from build123d import *

# Parameters (mm, degrees)
SKETCH_R             = 1.5
PAD_DEPTH            = 35
PAD001_DEPTH         = 0.5
SKETCH002_R          = 1.5
PAD002_DEPTH         = 19
PAD003_DEPTH         = 0.5
POLARPATTERN_COUNT   = 2
POLARPATTERN_ANGLE   = 90
SKETCH004_R          = 10
PAD004_DEPTH         = 10
SKETCH006_W          = 5.388718
SKETCH006_H          = 19
SKETCH006_W_2        = 5.907516
POCKET_DEPTH         = 5
SKETCH005_W          = 53.248554
SKETCH005_H          = 72.779518
SKETCH005_W_2        = 13.520593
SKETCH005_H_2        = 41.716759
POCKET001_DEPTH      = 10.001
POCKET001_DEPTH_BACK = -10.001


with BuildPart() as part:
    # Sketch → Pad (new body)
    with BuildSketch(Plane.XY):
        Circle(SKETCH_R)
    extrude(amount=PAD_DEPTH)

    # Sketch001 → Pad001 (join, symmetric)
    with BuildSketch(Plane.XZ):
        Polygon((-3.25, 0), (3.25, 0), (3.25, 1.5), (1.083333, 4.5), (3.25, 7.5), (3.25, 9), (-3.25, 9), (-3.25, 7.5), (-1.083333, 4.5), (-3.25, 1.5), align=None)
    extrude(amount=PAD001_DEPTH, both=True)

    # Sketch002 → Pad002 (join)
    with BuildSketch(Plane.XY):
        Circle(SKETCH002_R)
    extrude(amount=-PAD002_DEPTH)

    # Sketch003 → Pad003 (join, symmetric)
    with BuildSketch(Plane.XZ):
        Polygon((-3.4, -19), (3.4, -19), (3.4, -9), (0, 2), (-3.4, -9), align=None)
    pad003 = extrude(amount=PAD003_DEPTH, both=True)

    # PolarPattern: Pad003 ×2 about axis
    polarpattern_axis = Axis((0, 0, 0), (0, 0, 1))
    for i in range(1, POLARPATTERN_COUNT):
        add(pad003.rotate(polarpattern_axis, i * POLARPATTERN_ANGLE / (POLARPATTERN_COUNT - 1)))

    # Sketch004 → Pad004 (join)
    with BuildSketch(Plane.XY.offset(-19)):
        Circle(SKETCH004_R)
    extrude(amount=-PAD004_DEPTH)

    # Sketch006 → Pocket (cut, symmetric)
    with BuildSketch(Plane.YZ):
        with Locations((5.194359, -9.5)):
            Rectangle(SKETCH006_W, SKETCH006_H)
        with Locations((-5.453758, -9.5)):
            Rectangle(SKETCH006_W_2, SKETCH006_H)
    extrude(amount=POCKET_DEPTH, both=True, mode=Mode.SUBTRACT)

    # Sketch005 → Pocket001 (cut, two sides)
    with BuildSketch(Plane.XZ) as pocket001_sk:
        with Locations((-0.717024, -0.672455)):
            Rectangle(SKETCH005_W, SKETCH005_H)
        with Locations((0.133193, -10.244297)):
            Rectangle(SKETCH005_W_2, SKETCH005_H_2, mode=Mode.SUBTRACT)
    extrude(amount=-POCKET001_DEPTH, mode=Mode.SUBTRACT)
    extrude(pocket001_sk.sketch, amount=-POCKET001_DEPTH_BACK, mode=Mode.SUBTRACT)


solid = part.part
Design review of the part built by this model. Coordinates are the model's own, in mm. A direction names the side the tool comes from. Round coordinates to 2 decimals unless told otherwise and drop trailing zeros. Write each loop counter-clockwise with the first axis right and the second up, starting at its lowest first coordinate (ties: lowest second). Pieces come first, ordered by that corner, then holes. Notation, with made-up numbers: (8, -37.5) - (51, -37.5) arc R24 cw to (51, -20.5) - close; hole circle Ø5 at (8, 84). An arc over 180 degrees is marked (long way). Return JSON: item names as keys, results as strings. Group by question number.
Item 1: We need section B-B on x = 0. Write out the cut boundary in (y, z).
Item 2: Machinability: for faces 4 (the face through (2, -0.5, -12)), 5 (the face through (-3.4, 0, -14)), 6 (the face through (0, -2.5, -13)), 7 (the face through (-2, 0.5, 7)), 8 (the face through (0, 2.5, -13)), which of the approach directions +Z, -Z, +X, -X, +Y, -Y give a long, thin tool a straight path to every point of the face, cutting with its end or side? Answer none if there is none.
Item 3: For probe 1 along Z at (x, y) = (0.75, -1.5); probe 2 along Y at (x, z) = (3.25, -12); probe 3 along X at (y, z) = (-9, -20), list the stretches that pass through material, from the lowest coordinate up. Write a range as [from, to].
Item 4: We need section C-C on y = 3.75. Write out the cut boundary in (x, z), and give its area (3 significant figures).
Item 5: We need section A-A on z = -13.5. Write out the cut boundary in (x, y).
Item 6: We need section D-D on z = 1. Write out the cut boundary in (x, y), and give its area (3 significant figures).
Item 7: Insertion check: P1, Ø0.5, axis at x = 0, z = -12, coming from the +Y side; P2, Ø0.6, axis at x = 2.5, z = 7, coming from the +Y side; P3, Ø2, axis at x = 2, z = 6, coming from the -Y side. Each pin has a flat end and moves straight along its axis. Give the tip position at first contact, or say it passes through.
Item 8: The part is to be moulded in two halves that separate along Z. For faces 1 (the face through (2, 0.5, 2)), 2 (the face through (-2, 0, 9)), 3 (the face through (-2.32, -0.01, 2.79)), say which applies: pulls with the +Z half, pulls with the -Z half, needs draft (parallel to the pull), parting line crosses it, or undercut.
Model answer:
{
 "1": {"outline": "(-10, -29) - (10, -29) - (10, -19) - (2.5, -19) - (2.5, -6.09) - (1.5, -2.85) - (1.5, 10.61) - (-1.5, 10.61) - (-1.5, -2.85) - (-2.5, -6.09) - (-2.5, -19) - (-10, -19) - close"},
 "2": {"face 4": "+Z, +X, -Y", "face 5": "+Z, -X, +Y, -Y", "face 6": "+Z, +X, -X, -Y", "face 7": "+Z, -X, +Y", "face 8": "+Z, +X, -X, +Y"},
 "3": {"probe 1": "z = [-29, -19]", "probe 2": "y = [-0.5, 0.5]", "probe 3": "x = [-4.36, 4.36]"},
 "4": {"outline": "(-6.63, -29) - (6.89, -29) - (6.89, -19) - (-6.63, -19) - close", "area": "135 mm²"},
 "5": {"outline": "(-3.4, -0.5) - (-1.41, -0.5) arc R1.5 ccw to (-0.5, -1.41) - (-0.5, -2.5) - (0.5, -2.5) - (0.5, -1.41) arc R1.5 ccw to (1.41, -0.5) - (3.4, -0.5) - (3.4, 0.5) - (1.41, 0.5) arc R1.5 ccw to (0.5, 1.41) - (0.5, 2.5) - (-0.5, 2.5) - (-0.5, 1.41) arc R1.5 ccw to (-1.41, 0.5) - (-3.4, 0.5) - close"},
 "6": {"outline": "(-3.25, -0.5) - (-1.41, -0.5) arc R1.5 ccw to (1.41, -0.5) - (3.25, -0.5) - (3.25, 0.5) - (1.41, 0.5) arc R1.5 ccw to (-1.41, 0.5) - (-3.25, 0.5) - close", "area": "10.6 mm²"},
 "7": {"P1": "stops at y = 2.5", "P2": "stops at y = 0.5", "P3": "stops at y = -1.12"},
 "8": {"face 1": "needs draft", "face 2": "pulls with the +Z half", "face 3": "undercut"}
}
